from build123d import *

# Parameters (mm, degrees)
SALIENTE_EXTRUIR1_DEPTH  = 58.05
REDONDEO1_R              = 20
REDONDEO2_R              = 20
REDONDEO3_R              = 17
REDONDEO4_R              = 17
CAVIDAD1_START           = -47
CAVIDAD1_DEPTH           = 51
CROQUIS8_W               = 12
CROQUIS8_H               = 3
SALIENTE_EXTRUIR2_DEPTH  = 38
CROQUIS9_R               = 2.25
CORTAR_EXTRUIR6_DEPTH    = 135.588949923
SALIENTE_EXTRUIR3_REACH  = 146.947
CROQUIS11_W              = 20
CROQUIS11_H              = 3
CROQUIS12_W              = 69.238292886
CROQUIS12_H              = 3
CORTAR_EXTRUIR7_DEPTH    = 1
CROQUIS15_R              = 1.75
CORTAR_EXTRUIR10_DEPTH   = 5
REDONDEO5_R              = 7
REDONDEO6_R              = 3
CROQUIS18_R              = 11
CORTAR_EXTRUIR12_DEPTH   = 146.081609054
CROQUIS19_R              = 13.25
CROQUIS19_R_2            = 11
SALIENTE_EXTRUIR4_DEPTH  = 5
CROQUIS16_R              = 65
CORTAR_EXTRUIR11_DEPTH   = 145.946782753
SALIENTE_EXTRUIR5_DEPTH  = 3
NERVIO8_START            = -1.125
NERVIO8_DEPTH            = 2.25
MATRIZC2_COUNT           = 6
REDONDEO6_OF_SIMETR_A1_R = 3
REDONDEO7_R              = 10
REDONDEO8_R              = 10
REDONDEO9_R              = 6
CORTAR_EXTRUIR14_DEPTH   = 145.946782753
REDONDEO10_R             = 5


with BuildPart() as part:
    # Croquis1 → Saliente-Extruir1 (new, symmetric)
    with BuildSketch(Plane(origin=(0, 0, 0), x_dir=(0, 0, -1), z_dir=(1, 0, 0))):
        Polygon((0, 0), (0, 67.196152423), (28.732050808, 116.961524227), (47, 116.961524227), (47, 119.961524227), (27, 119.961524227), (-3, 68), (-3, 0), align=None)
    extrude(amount=SALIENTE_EXTRUIR1_DEPTH, both=True)

    # Redondeo1
    redondeo1_edges = [part.edges().sort_by_distance(p)[0] for p in [
        (0, 68, 3),
    ]]
    fillet(redondeo1_edges, radius=REDONDEO1_R)

    # Redondeo2
    redondeo2_edges = [part.edges().sort_by_distance(p)[0] for p in [
        (0, 119.961524227, -27),
    ]]
    fillet(redondeo2_edges, radius=REDONDEO2_R)

    # Redondeo3
    redondeo3_edges = [part.edges().sort_by_distance(p)[0] for p in [
        (0, 116.961524227, -28.732050808),
    ]]
    fillet(redondeo3_edges, radius=REDONDEO3_R)

    # Redondeo4
    redondeo4_edges = [part.edges().sort_by_distance(p)[0] for p in [
        (0, 67.196152423, 0),
    ]]
    fillet(redondeo4_edges, radius=REDONDEO4_R)

    # Cavidad1: read off the stored shape, not the designer's step
    # Cavidad1 outline → Cavidad1 (cut)
    with BuildSketch(Plane.XY.offset(CAVIDAD1_START)):
        with BuildLine():
            Line((58.05, 0), (58.05, 119.961524227))
            Line((58.05, 119.961524227), (-5.55, 119.961524227))
            Line((-5.55, 119.961524227), (-5.55, 116.961524227))
            Line((-5.55, 116.961524227), (5.123846837, 116.961524227))
            ThreePointArc((5.123846837, 116.961524227), (12.308357287, 115.368756607), (18.14660237, 110.888913592))
            Line((18.14660237, 110.888913592), (51.073651347, 71.647984679))
            ThreePointArc((51.073651347, 71.647984679), (54.025670368, 66.534937751), (55.050895814, 60.720595315))
            Line((55.050895814, 60.720595315), (55.050895814, 0))
            Line((55.050895814, 0), (58.05, 0))
        make_face()
    extrude(amount=CAVIDAD1_DEPTH, mode=Mode.SUBTRACT)

    # Croquis8 → Saliente-Extruir2 (add)
    with BuildSketch(Plane(origin=(0, 0, 0), x_dir=(-1, 0, 0), z_dir=(0, 0, -1))):
        with Locations((-47.050895814, 6.5)):
            Rectangle(CROQUIS8_W, CROQUIS8_H)
    saliente_extruir2 = extrude(amount=SALIENTE_EXTRUIR2_DEPTH)

    # Croquis9 → Cortar-Extruir6 (cut, through all)
    with BuildSketch(Plane(origin=(0, 8, 0), x_dir=(1, 0, 0), z_dir=(0, 1, 0))):
        with Locations(Location((47.050895814, 33, 0), (0, 0, 180))):
            Circle(CROQUIS9_R)
    cortar_extruir6 = extrude(amount=-CORTAR_EXTRUIR6_DEPTH, mode=Mode.SUBTRACT)

    # Saliente-Extruir3: up to this plane
    saliente_extruir3_end = Plane(origin=(58.05, 67.196152423, 0), z_dir=(0, 0.49999999999999767, 0.86602540378444))
    # Croquis11 → Saliente-Extruir3 (add, up to the surface)
    with BuildSketch(Plane(origin=(0, 0, -54), x_dir=(-1, 0, 0), z_dir=(0, 0, -1)), mode=Mode.PRIVATE) as saliente_extruir3_sk1:
        with Locations((28.05, 92.461524227)):
            Rectangle(CROQUIS11_W, CROQUIS11_H)
    saliente_extruir3_tool1 = split(extrude(saliente_extruir3_sk1.sketch, amount=-SALIENTE_EXTRUIR3_REACH, mode=Mode.PRIVATE), bisect_by=saliente_extruir3_end, keep=Keep.BOTH, mode=Mode.PRIVATE)
    add(saliente_extruir3_tool1.solids().sort_by_distance((-28.05, 92.461524, -54))[0])

    # Croquis12 → Cortar-Extruir7 (cut)
    with BuildSketch(Plane.XZ):
        with Locations((20.431749371, 1.5)):
            Rectangle(CROQUIS12_W, CROQUIS12_H)
    extrude(amount=-CORTAR_EXTRUIR7_DEPTH, mode=Mode.SUBTRACT)

    # Croquis15 → Cortar-Extruir10 (cut)
    with BuildSketch(Plane.XZ.offset(-90.961524227)):
        with Locations(Location((-28.049104186, -49.5, 0), (0, 0, 270))):
            Circle(CROQUIS15_R)
    extrude(amount=-CORTAR_EXTRUIR10_DEPTH, mode=Mode.SUBTRACT)

    # Redondeo5
    redondeo5_edges = [part.edges().sort_by_distance(p)[0] for p in [
        (-18.05, 92.461524227, -54),
        (-38.05, 92.461524227, -54),
    ]]
    fillet(redondeo5_edges, radius=REDONDEO5_R)

    # Redondeo6
    redondeo6_edges = [part.edges().sort_by_distance(p)[0] for p in [
        (53.050895814, 6.5, -38),
        (41.050895814, 6.5, -38),
    ]]
    fillet(redondeo6_edges, radius=REDONDEO6_R)

    # Croquis18 → Cortar-Extruir12 (cut, through all)
    with BuildSketch(Plane(origin=(0, 18.299038106, 31.694863729), x_dir=(1, 0, 0), z_dir=(0, 0.4999999999999976, 0.86602540378444))):
        with Locations(Location((7.567578046, 85.748711306, 0), (0, 0, 270))):
            Circle(CROQUIS18_R)
    extrude(amount=-CORTAR_EXTRUIR12_DEPTH, mode=Mode.SUBTRACT)

    # Croquis19 → Saliente-Extruir4 (add)
    with BuildSketch(Plane(origin=(0, 16.799038106, 29.096787517), x_dir=(-1, 0, 0), z_dir=(0, -0.4999999999999977, -0.8660254037844399))):
        with Locations(Location((-7.567578046, 85.748711306, 0), (0, 0, 270))):
            Circle(CROQUIS19_R)
        with Locations(Location((-7.567578046, 85.748711306, 0), (0, 0, 270))):
            Circle(CROQUIS19_R_2, mode=Mode.SUBTRACT)
    extrude(amount=SALIENTE_EXTRUIR4_DEPTH)

    # Croquis16 → Cortar-Extruir11 (cut, through all)
    with BuildSketch(Plane.XY.offset(3)):
        with Locations((-45.071920691, 22.721524227)):
            Circle(CROQUIS16_R)
    extrude(amount=-CORTAR_EXTRUIR11_DEPTH, mode=Mode.SUBTRACT)

    # Croquis25 → Saliente-Extruir5 (add)
    with BuildSketch(Plane.XZ.offset(-90.961524227)):
        Polygon((-38.05, -13.720943809), (-45.254421175, -13.720943809), (-38.05, -47), align=None)
        Polygon((-10.845578825, -13.720943809), (-18.05, -47), (-18.05, -13.720943809), align=None)
    extrude(amount=-SALIENTE_EXTRUIR5_DEPTH)

    # Nervio8: read off the stored shape, not the designer's step
    # Nervio8 outline → Nervio8 (add)
    with BuildSketch(Plane(origin=(46.658144676, 40.407138583, -23.329072338), x_dir=(-0.707106781186543, 0.6123724356957992, -0.35355339059327456), z_dir=(-0.7071067811865521, -0.6123724356957916, 0.35355339059326985)).offset(NERVIO8_START)):
        Polygon((42.080255309, -28.598076211), (42.032409489, -28.598076211), (34.032409489, -33.598076211), (42.080255309, -33.598076211), align=None)
    nervio8 = extrude(amount=NERVIO8_DEPTH)

    # MatrizC2: Nervio8 ×6 about axis
    matrizc2_axis = Axis((7.567578046, 74.260562333, -42.874355653), (0, -0.49999999999999767, -0.86602540378444))
    for i in range(1, MATRIZC2_COUNT):
        add(nervio8.rotate(matrizc2_axis, i * 360 / MATRIZC2_COUNT))

    # Simetría1: Saliente-Extruir2, Cortar-Extruir6 across plane
    add(saliente_extruir2.mirror(Plane(origin=(37.445895814, 0, 0), x_dir=(0, 0, 1), z_dir=(1, 0, 0))))
    add(cortar_extruir6.mirror(Plane(origin=(37.445895814, 0, 0), x_dir=(0, 0, 1), z_dir=(1, 0, 0))), mode=Mode.SUBTRACT)

    # Redondeo6 of Simetría1
    redondeo6_of_simetr_a1_edges = [part.edges().sort_by_distance(p)[0] for p in [
        (21.840895814, 6.5, -38),
        (33.840895814, 6.5, -38),
    ]]
    fillet(redondeo6_of_simetr_a1_edges, radius=REDONDEO6_OF_SIMETR_A1_R)

    # Redondeo7
    # the kernel refuses this fillet: 10 mm, written as the material it adds along each edge
    with BuildSketch(Plane(origin=(21.050895814, 5, 0), x_dir=(0, -1, 0), z_dir=(1, 0, 0))) as redondeo7_piece_1_section:
        with BuildLine():
            CenterArc((10, 8), REDONDEO7_R, 180, 53.130102354)
            Line((0, 8), (-0.2, 8))
            Line((-0.2, 8), (-0.2, 0))
            Line((-0.2, 0), (0, -0.2))
            ThreePointArc((0, -0.2), (2, -0.2), (3.88, -0.16))
            Line((3.88, -0.16), (4, 0))
        make_face()
    redondeo7_piece_1 = extrude(amount=32, mode=Mode.PRIVATE)
    redondeo7_piece_1 = split(redondeo7_piece_1, bisect_by=Plane(origin=(21.840895814, 5, 0), z_dir=(1, 0, 0)), keep=Keep.TOP, mode=Mode.PRIVATE)
    redondeo7_piece_1 = split(redondeo7_piece_1, bisect_by=Plane(origin=(33.840895814, 5, 0), z_dir=(-1, 0, 0)), keep=Keep.TOP, mode=Mode.PRIVATE)
    add(redondeo7_piece_1)
    with BuildSketch(Plane(origin=(41.050895814, 5, 0), x_dir=(0, -1, 0), z_dir=(1, 0, 0))) as redondeo7_piece_2:
        with BuildLine():
            CenterArc((10, 8), REDONDEO7_R, 180, 53.130102354)
            Line((0, 8), (-0.2, 8))
            Line((-0.2, 8), (-0.2, 0))
            Line((-0.2, 0), (0, -0.2))
            ThreePointArc((0, -0.2), (2, -0.2), (3.88, -0.16))
            Line((3.88, -0.16), (4, 0))
        make_face()
    extrude(amount=12)
    with BuildSketch(Plane(origin=(53.840895814, 5, 0), x_dir=(0, -1, 0), z_dir=(-1, 0, 0))) as redondeo7_piece_3_section:
        with BuildLine():
            CenterArc((10, -8), REDONDEO7_R, 126.869897646, 53.130102354)
            Line((0, -8), (-0.2, -8))
            Line((-0.2, -8), (-0.2, 0))
            Line((-0.2, 0), (0, 0.2))
            ThreePointArc((0, 0.2), (2, 0.2), (3.88, 0.16))
            Line((3.88, 0.16), (4, 0))
        make_face()
    redondeo7_piece_3 = extrude(amount=32, mode=Mode.PRIVATE)
    redondeo7_piece_3 = split(redondeo7_piece_3, bisect_by=Plane(origin=(53.050895814, 5, 0), z_dir=(-1, 0, 0)), keep=Keep.TOP, mode=Mode.PRIVATE)
    redondeo7_piece_3 = split(redondeo7_piece_3, bisect_by=Plane(origin=(41.050895814, 5, 0), z_dir=(1, 0, 0)), keep=Keep.TOP, mode=Mode.PRIVATE)
    add(redondeo7_piece_3)
    with BuildSketch(Plane(origin=(33.840895814, 5, 0), x_dir=(0, -1, 0), z_dir=(-1, 0, 0))) as redondeo7_piece_4:
        with BuildLine():
            CenterArc((10, -8), REDONDEO7_R, 126.869897646, 53.130102354)
            Line((0, -8), (-0.2, -8))
            Line((-0.2, -8), (-0.2, 0))
            Line((-0.2, 0), (0, 0.2))
            ThreePointArc((0, 0.2), (2, 0.2), (3.88, 0.16))
            Line((3.88, 0.16), (4, 0))
        make_face()
    extrude(amount=12)

    # Redondeo8
    redondeo8_edges = [part.edges().sort_by_distance(p)[0] for p in [
        (47.050895814, 8, 0),
        (27.840895814, 8, 0),
    ]]
    fillet(redondeo8_edges, radius=REDONDEO8_R)

    # Redondeo9
    redondeo9_edges = [part.edges().sort_by_distance(p)[0] for p in [
        (-28.05, 93.961524227, -15.452994616),
    ]]
    fillet(redondeo9_edges, radius=REDONDEO9_R)

    # Croquis31 → Cortar-Extruir14 (cut, through all)
    with BuildSketch(Plane.XY.offset(3)):
        with BuildLine():
            Line((16.191244305, 1), (19.497703143, 1))
            Line((19.497703143, 1), (19.844268253, 19.421764692))
            ThreePointArc((19.844268253, 19.421764692), (18.686590065, 10.078253042), (16.191244305, 1))
        make_face()
    extrude(amount=-CORTAR_EXTRUIR14_DEPTH, mode=Mode.SUBTRACT)

    # Redondeo10
    redondeo10_edges = [part.edges().sort_by_distance(p)[0] for p in [
        (-28.05, 90.961524227, -13.720943809),
    ]]
    fillet(redondeo10_edges, radius=REDONDEO10_R)


solid = part.part
Model file for the job. Use its own axes, mm. A direction names the side the tool comes from. Coordinates: 2 decimals unless noted, no trailing zeros. Write each loop counter-clockwise with the first axis right and the second up, starting at its lowest first coordinate (ties: lowest second). Pieces come first, ordered by that corner, then holes. Notation, with made-up numbers: (79, -33.5) - (112, -33.5) arc R25 ccw to (112, -0.5) - close; hole circle Ø1 at (-10, 16). An arc over 180 degrees is marked (long way). Write each question's results on one line, items separated by ' | '. Start each with the question number.
1) Probe line 1 along X through (y, z) = (10, -0.5); line 2 along Z through (x, y) = (27.5, 32); line 3 along Y through (x, z) = (45.5, -5.5). List the from-to ranges inside material, lowest first. Write a range as from..to.
2) Cut at C-C (y = 10.5). Write the cut outline in (x, z).
3) 3-axis set-ups, long thin cutter, end or side, ignore diameter. For faces 1 (the face through (-27.52, 92.44, -51.17)), 2 (the face through (27.92, 10.85, -3.01)), 3 (the face through (4.06, 100.892, -22.301)): which of +Z, -Z, +X, -X, +Y, -Y reach the whole face in a straight line?
4) Cut at B-B (z = -49.5). Write the cut outline in (x, y).
5) Cut at D-D (y = 50). Write the cut outline in (x, z), then the cut area to 3 significant figures.
6) Cut at A-A (z = -33). Write the cut outline in (x, y).
7) Mould opens along X. For faces 4 (the face through (33.841, 6, -14)), 5 (the face through (19.32, 81.55, -9.93)), 6 (the face through (22.7, 6.5, -37.1)), 7 (the face through (-28, 93.962, -40)) say: pulls with the +X half, pulls with the -X half, needs draft (parallel to the pull), parting line crosses it, or undercut.
8) Flat gauge pins, fed straight in: P1, Ø2.5, axis at x = -36.5, y = 118.5, coming from the -Z side; P2, Ø6, axis at x = 25.5, z = -23, coming from the -Y side; P3, Ø3, axis at x = -2, z = -34.5, coming from the +Y side; P4, Ø3.5, axis at x = 47.05, z = -33, coming from the +Y side. Where does each tip first touch, or does it go through?
Returned:
1) line 1: 21.84..33.84, 41.05..53.05 | line 2: 0..3 | line 3: 4.68..9.07, 76.72..78.29
2) outline: (19.68, 0) - (21.84, 0) - (21.84, -3.39) - (33.84, -3.39) - (33.84, 0) - (41.05, 0) - (41.05, -3.39) - (53.05, -3.39) - (53.05, 0) - (55.05, 0) - (55.05, 3) - (19.68, 3) - close
3) face 1: +Y, -Y | face 2: -Z, +X, -X | face 3: -Z
4) outline: (-37.59, 90.96) - (-29.8, 90.96) - (-29.8, 93.96) - (-37.59, 93.96) - close; (-26.3, 90.96) - (-18.51, 90.96) - (-18.51, 93.96) - (-26.3, 93.96) - close
5) outline: (13.93, 0) - (55.05, 0) - (55.05, 3) - (13.93, 3) - close | area: 123 mm^2
6) outline: (-58.05, 116.03) - (10.67, 116.03) arc R17 ccw to (5.12, 116.96) - (-5.55, 116.96) - (-5.55, 119.18) - (-58.05, 119.18) - close; (-41.08, 90.96) - (-15.02, 90.96) - (-15.02, 93.96) - (-41.08, 93.96) - close; (21.84, 5) - (25.59, 5) - (25.59, 8) - (21.84, 8) - close; (30.09, 5) - (33.84, 5) - (33.84, 8) - (30.09, 8) - close; (41.05, 5) - (44.8, 5) - (44.8, 8) - (41.05, 8) - close; (49.3, 5) - (53.05, 5) - (53.05, 8) - (49.3, 8) - close
7) face 4: undercut | face 5: pulls with the +X half | face 6: pulls with the -X half | face 7: needs draft
8) P1: z = -47 | P2: y = 5 | P3: y = 116.96 | P4: through
